```python
from build123d import *

# Parameters (mm, degrees)
EXTRUDE_1_DEPTH      = 12
CUT_EXTRUDE_1_DEPTH  = 12
SKETCH_3_R           = 2
CUT_EXTRUDE_2_DEPTH  = 12
CUT_EXTRUDE_3_DEPTH  = 1
SKETCH_5_W           = 80
SKETCH_5_H           = 4
CUT_EXTRUDE_4_DEPTH  = 20
EXTRUDE_2_DEPTH      = 1
SKETCH_7_W           = 0.2
SKETCH_7_H           = 8
CUT_EXTRUDE_5_DEPTH  = 1
SKETCH_8_R           = 2
EXTRUDE_3_DEPTH      = 4
SKETCH_9_W           = 80
SKETCH_9_H           = 9
CUT_EXTRUDE_6_DEPTH  = 14
SKETCH_10_W          = 9.44
SKETCH_10_H          = 1
CUT_EXTRUDE_7_DEPTH  = 14
SKETCH_11_W          = 9.44
SKETCH_11_H          = 1
EXTRUDE_4_DEPTH      = 8
CUT_EXTRUDE_8_DEPTH  = 8
SKETCH_13_W          = 80
SKETCH_13_H          = 3
EXTRUDE_5_DEPTH      = 7
SKETCH_14_R          = 1.6
EXTRUDE_7_DEPTH      = 3
SKETCH_16_W          = 3
SKETCH_16_H          = 4
EXTRUDE_8_DEPTH      = 80
SKETCH_17_R          = 1.55
CUT_EXTRUDE_11_DEPTH = 7
SKETCH_21_R          = 2
CUT_EXTRUDE_12_DEPTH = 7
EXTRUDE_9_DEPTH      = 4
SKETCH_23_W          = 3
SKETCH_23_H          = 4
CUT_EXTRUDE_13_DEPTH = 200
CUT_EXTRUDE_15_DEPTH = 5
SKETCH_25_W          = 9.44
SKETCH_25_H          = 4
CUT_EXTRUDE_16_DEPTH = 5
SKETCH_26_W          = 9.44
SKETCH_26_H          = 4
EXTRUDE_10_DEPTH     = 2
SKETCH_27_W          = 9.44
SKETCH_27_H          = 4
EXTRUDE_11_DEPTH     = 1
SKETCH_28_W          = 5
SKETCH_28_H          = 14
CUT_EXTRUDE_17_DEPTH = 1
SKETCH_29_W          = 5
SKETCH_29_H          = 4
EXTRUDE_12_DEPTH     = 1


with BuildPart() as part:
    # 草图1 → 凸台-拉伸1 (new body)
    with BuildSketch(Plane(origin=(0, 0, 0), x_dir=(1, 0, 0), z_dir=(0, 1, 0))):
        Polygon((-40, -6), (0, -6), (40, -6), (40, 0), (40, 6), (0, 6), (-36, 6), (-40, 6), align=None)
    extrude(amount=EXTRUDE_1_DEPTH)

    # 草图2 → 切除-拉伸1 (cut)
    with BuildSketch(Plane.XY.offset(6)):
        Polygon((-28, 0), (0, 0), (28, 0), (28, 4), (28, 8), (-28, 8), (-28, 4), align=None)
        Polygon((-40, 4), (-32, 4), (-32, 8), (-32, 12), (-40, 12), align=None)
        Polygon((32, 8), (32, 4), (40, 4), (40, 12), (32, 12), align=None)
    extrude(amount=-CUT_EXTRUDE_1_DEPTH, mode=Mode.SUBTRACT)

    # 草图3 → 切除-拉伸2 (cut)
    with BuildSketch(Plane(origin=(0, 12, 0), x_dir=(1, 0, 0), z_dir=(0, 1, 0))):
        with BuildLine():
            Line((-40, 6), (-40, 4))
            ThreePointArc((-40, 4), (-39.414213562, 5.414213562), (-38, 6))
            Line((-38, 6), (-40, 6))
        make_face()
        with Locations(Location((-36, 2, 0), (0, 0, 270))):
            Circle(SKETCH_3_R)
        with BuildLine():
            ThreePointArc((40, 4), (39.414213562, 5.414213562), (38, 6))
            Line((38, 6), (40, 6))
            Line((40, 6), (40, 4))
        make_face()
        with Locations(Location((36, 2, 0), (0, 0, 270))):
            Circle(SKETCH_3_R)
    extrude(amount=-CUT_EXTRUDE_2_DEPTH, mode=Mode.SUBTRACT)

    # 草图4 → 切除-拉伸3 (cut)
    with BuildSketch(Plane(origin=(0, 12, 0), x_dir=(1, 0, 0), z_dir=(0, 1, 0))):
        Polygon((-21.1, 0), (-21.1, 6), (-16.6, 6), (-12.1, 6), (12.08, 6), (16.6, 6), (21.12, 6), (21.12, -1), (21.12, -6), (16.6, -6), (12.08, -6), (12.08, -1), (12.08, 0), (-12.1, 0), (-12.1, -6), (-16.6, -6), (-21.1, -6), align=None)
    extrude(amount=-CUT_EXTRUDE_3_DEPTH, mode=Mode.SUBTRACT)

    # 草图5 → 切除-拉伸4 (cut)
    with BuildSketch(Plane(origin=(0, 12, 0), x_dir=(1, 0, 0), z_dir=(0, 1, 0))):
        with Locations((0, -4)):
            Rectangle(SKETCH_5_W, SKETCH_5_H)
    extrude(amount=-CUT_EXTRUDE_4_DEPTH, mode=Mode.SUBTRACT)

    # 草图6 → 凸台-拉伸2 (add)
    with BuildSketch(Plane(origin=(0, 12, 0), x_dir=(1, 0, 0), z_dir=(0, 1, 0))):
        Polygon((12.08, 0), (12.08, 6), (-21.1, 6), (-21.1, -2), (-12.1, -2), (-12.1, 0), align=None)
    extrude(amount=-EXTRUDE_2_DEPTH)

    # 草图7 → 切除-拉伸5 (cut)
    with BuildSketch(Plane(origin=(0, 12, 0), x_dir=(1, 0, 0), z_dir=(0, 1, 0))):
        with Locations((21.22, 2)):
            Rectangle(SKETCH_7_W, SKETCH_7_H)
        with Locations((11.98, 2)):
            Rectangle(SKETCH_7_W, SKETCH_7_H)
    extrude(amount=-CUT_EXTRUDE_5_DEPTH, mode=Mode.SUBTRACT)

    # 草图8 → 凸台-拉伸3 (add)
    # profile 1 of 2: a face of its own
    with BuildSketch(Plane(origin=(0, 12, 0), x_dir=(1, 0, 0), z_dir=(0, 1, 0))):
        with BuildLine():
            Line((-32, -2), (-40, -2))
            Line((-40, -2), (-40, 4))
            ThreePointArc((-40, 4), (-39.414213562, 5.414213562), (-38, 6))
            Line((-38, 6), (-32, 6))
            Line((-32, 6), (-32, -2))
        make_face()
        with Locations(Location((-36, 2, 0), (0, 0, 270))):
            Circle(SKETCH_8_R, mode=Mode.SUBTRACT)
    # profile 2 of 2: a face of its own
    with BuildSketch(Plane(origin=(0, 12, 0), x_dir=(1, 0, 0), z_dir=(0, 1, 0))):
        with BuildLine():
            Line((32, -2), (40, -2))
            Line((40, -2), (40, 4))
            ThreePointArc((40, 4), (39.414213562, 5.414213562), (38, 6))
            Line((38, 6), (32, 6))
            Line((32, 6), (32, -2))
        make_face()
        with Locations(Location((36, 2, 0), (0, 0, 270))):
            Circle(SKETCH_8_R, mode=Mode.SUBTRACT)
    extrude(amount=-EXTRUDE_3_DEPTH)

    # 草图9 → 切除-拉伸6 (cut)
    with BuildSketch(Plane.XY.offset(2)):
        with Locations((0, 4.5)):
            Rectangle(SKETCH_9_W, SKETCH_9_H)
    extrude(amount=-CUT_EXTRUDE_6_DEPTH, mode=Mode.SUBTRACT)

    # 草图10 → 切除-拉伸7 (cut)
    with BuildSketch(Plane(origin=(0, 0, -6), x_dir=(-1, 0, 0), z_dir=(0, 0, -1))):
        with Locations((-16.6, 9.5)):
            Rectangle(SKETCH_10_W, SKETCH_10_H)
    extrude(amount=-CUT_EXTRUDE_7_DEPTH, mode=Mode.SUBTRACT)

    # 草图11 → 凸台-拉伸4 (add)
    with BuildSketch(Plane(origin=(0, 0, -6), x_dir=(-1, 0, 0), z_dir=(0, 0, -1))):
        with Locations((-16.6, 11.5)):
            Rectangle(SKETCH_11_W, SKETCH_11_H)
    extrude(amount=-EXTRUDE_4_DEPTH)

    # 草图12 → 切除-拉伸8 (cut)
    with BuildSketch(Plane.XZ.offset(-9)):
        with BuildLine():
            ThreePointArc((21.05, -2.72), (18.302941274, 1.39126392), (13.453374824, 0.426625176))
            Line((13.453374824, 0.426625176), (19.746625176, -5.866625176))
            ThreePointArc((19.746625176, -5.866625176), (20.71126392, -4.422941274), (21.05, -2.72))
        make_face()
        with BuildLine():
            Line((19.746625176, -5.866625176), (13.453374824, 0.426625176))
            ThreePointArc((13.453374824, 0.426625176), (13.453374824, -5.866625176), (19.746625176, -5.866625176))
        make_face()
    extrude(amount=-CUT_EXTRUDE_8_DEPTH, mode=Mode.SUBTRACT)

    # 草图13 → 凸台-拉伸5 (add)
    with BuildSketch(Plane(origin=(0, 12, 0), x_dir=(1, 0, 0), z_dir=(0, 1, 0))):
        with Locations((0, -3.5)):
            Rectangle(SKETCH_13_W, SKETCH_13_H)
    extrude(amount=-EXTRUDE_5_DEPTH)

    # 草图14 → 凸台-拉伸7 (add)
    with BuildSketch(Plane(origin=(0, 12, 0), x_dir=(1, 0, 0), z_dir=(0, 1, 0))):
        with BuildLine():
            Line((-40, -100), (-40, -5))
            Line((-40, -5), (40, -5))
            Line((40, -5), (40, -100))
            Line((40, -100), (40, -102))
            ThreePointArc((40, -102), (39.414213562, -103.414213562), (38, -104))
            Line((38, -104), (36, -104))
            Line((36, -104), (-36, -104))
            Line((-36, -104), (-38, -104))
            ThreePointArc((-38, -104), (-39.414213562, -103.414213562), (-40, -102))
            Line((-40, -102), (-40, -100))
        make_face()
        with Locations(Location((-36, -100, 0), (0, 0, 270))):
            Circle(SKETCH_14_R, mode=Mode.SUBTRACT)
        with Locations(Location((36, -100, 0), (0, 0, 270))):
            Circle(SKETCH_14_R, mode=Mode.SUBTRACT)
    extrude(amount=-EXTRUDE_7_DEPTH)

    # 草图16 → 凸台-拉伸8 (add)
    with BuildSketch(Plane.ZY.offset(40)):
        with Locations((94.5, 7)):
            Rectangle(SKETCH_16_W, SKETCH_16_H)
    extrude(amount=-EXTRUDE_8_DEPTH)

    # 草图17 → 切除-拉伸11 (cut)
    with BuildSketch(Plane(origin=(0, 12, 0), x_dir=(1, 0, 0), z_dir=(0, 1, 0))):
        with Locations(Location((1.6, -34, 0), (0, 0, 270))):
            Circle(SKETCH_17_R)
        with Locations(Location((31.6, -34, 0), (0, 0, 270))):
            Circle(SKETCH_17_R)
        with Locations(Location((31.6, -64, 0), (0, 0, 270))):
            Circle(SKETCH_17_R)
        with Locations(Location((1.6, -64, 0), (0, 0, 270))):
            Circle(SKETCH_17_R)
    extrude(amount=-CUT_EXTRUDE_11_DEPTH, mode=Mode.SUBTRACT)

    # 草图21 → 切除-拉伸12 (cut)
    with BuildSketch(Plane(origin=(0, 12, 0), x_dir=(1, 0, 0), z_dir=(0, 1, 0))):
        with Locations(Location((-36, -100, 0), (0, 0, 270))):
            Circle(SKETCH_21_R)
        with Locations(Location((36, -100, 0), (0, 0, 270))):
            Circle(SKETCH_21_R)
    extrude(amount=-CUT_EXTRUDE_12_DEPTH, mode=Mode.SUBTRACT)

    # 草图22 → 凸台-拉伸9 (add)
    with BuildSketch(Plane(origin=(0, 9, 0), x_dir=(-1, 0, 0), z_dir=(0, -1, 0))):
        Polygon((40, -49), (40, -50.5), (-40, -50.5), (-40, -49), (-40, -47.5), (40, -47.5), align=None)
        Polygon((40, -26.25), (40, -27.75), (-40, -27.75), (-40, -24.75), (40, -24.75), align=None)
        Polygon((-40, -71.75), (-40, -73.25), (40, -73.25), (40, -70.25), (-40, -70.25), align=None)
    extrude(amount=EXTRUDE_9_DEPTH)

    # 草图23 → 切除-拉伸13 (cut)
    with BuildSketch(Plane.ZY.offset(40)):
        with Locations((3.5, 7)):
            Rectangle(SKETCH_23_W, SKETCH_23_H)
    extrude(amount=-CUT_EXTRUDE_13_DEPTH, mode=Mode.SUBTRACT)

    # 草图24 → 切除-拉伸15 (cut)
    with BuildSketch(Plane.XZ.offset(-9)):
        Polygon((11.88, -2), (11.88, 2), (16.6, 2), (16.6, 12), (9.6, 12), (9.6, -2), align=None)
        Polygon((16.6, 12), (16.6, 2), (21.32, 2), (21.32, -2), (23.6, -2), (23.6, 12), align=None)
    extrude(amount=-CUT_EXTRUDE_15_DEPTH, mode=Mode.SUBTRACT)

    # 草图25 → 切除-拉伸16 (cut)
    with BuildSketch(Plane(origin=(0, 10, 0), x_dir=(-1, 0, 0), z_dir=(0, -1, 0))):
        with Locations((-16.6, 0)):
            Rectangle(SKETCH_25_W, SKETCH_25_H)
    extrude(amount=-CUT_EXTRUDE_16_DEPTH, mode=Mode.SUBTRACT)

    # 草图26 → 凸台-拉伸10 (add)
    with BuildSketch(Plane(origin=(0, 10, 0), x_dir=(-1, 0, 0), z_dir=(0, -1, 0))):
        with Locations((-16.6, 4)):
            Rectangle(SKETCH_26_W, SKETCH_26_H)
    extrude(amount=-EXTRUDE_10_DEPTH)

    # 草图27 → 凸台-拉伸11 (add)
    with BuildSketch(Plane.XZ.offset(-10)):
        with Locations((16.6, -4)):
            Rectangle(SKETCH_27_W, SKETCH_27_H)
    extrude(amount=EXTRUDE_11_DEPTH)

    # 草图28 → 切除-拉伸17 (cut)
    with BuildSketch(Plane.XZ.offset(-9)):
        with Locations((7.1, 5)):
            Rectangle(SKETCH_28_W, SKETCH_28_H)
        with Locations((26.1, 5)):
            Rectangle(SKETCH_28_W, SKETCH_28_H)
    extrude(amount=-CUT_EXTRUDE_17_DEPTH, mode=Mode.SUBTRACT)

    # 草图29 → 凸台-拉伸12 (add)
    with BuildSketch(Plane.XZ.offset(-10)):
        with Locations((7.1, 0)):
            Rectangle(SKETCH_29_W, SKETCH_29_H)
        with Locations((26.1, 10)):
            Rectangle(SKETCH_29_W, SKETCH_29_H)
        with Locations((26.1, 0)):
            Rectangle(SKETCH_29_W, SKETCH_29_H)
        with Locations((7.1, 10)):
            Rectangle(SKETCH_29_W, SKETCH_29_H)
    extrude(amount=EXTRUDE_12_DEPTH)


solid = part.part
```
Check sheet for the modelled part. Datum: model origin and axes. Units: mm. A direction names the side the tool comes from. Give positions to 0.01 mm unless a question says otherwise; leave off trailing zeros. Order: outer loops, then holes, each group sorted by start corner. A loop starts at its lowest first (then second) coordinate and runs counter-clockwise, first axis right, second up. Notation, with made-up numbers: (13, 45) -> (45, 45) arc R7 cw to (45, 50) -> close; hole circle Ø9 at (33, 84.25). An arc over 180 degrees is marked (long way). Use CSV: the item, a comma, the result in double quotes. Start each with the question number.
1) Sectioned sample at B-B, the plane y = 7.5. Record the boundary of the cut face in (x, z), plus the area to 3 significant figures.
2) Set-up check for faces 1 (the face through (1, 9, 100)), 2 (the face through (-1, 7, 27.75)), 3 (the face through (26, 10, 5)), 4 (the face through (23.6, 11, 5)): record each of +Z, -Z, +X, -X, +Y, -Y from which the full face is reachable in a straight line by a thin tool's end or side.
3) Material ranges on line 1 (X direction, y = 10.75, z = 64); line 2 (X direction, y = 10.55, z = 100); line 3 (Z direction, x = -24, y = 6.25), recorded low to high. Write a range as from..to.
4) Mould release check, pull along Z, two halves, no side actions. Record for faces 5 (the face through (2.066, 10.521, 35.478)), 6 (the face through (-1, 11, -6)), 7 (the face through (1, 12, 48)): released by +Z, released by -Z, zero draft, split by the parting line, or undercut.
5) Sectioned sample at C-C, the plane x = 14.5. Record the boundary of the cut face in (y, z).
6) Sectioned sample at D-D, the plane x = 1.6. Record the boundary of the cut face in (y, z).
7) Sectioned sample at A-A, the plane z = 34. Record the boundary of the cut face in (x, y), plus the area to 3 significant figures.
8) Go/stop test with flat-tipped pins: P1, Ø1.2, axis at x = -14, y = 6.5, coming from the -Z side; P2, Ø10, axis at x = 11.5, z = 86.5, coming from the -Y side; P3, Ø3, axis at x = 10, y = 6.5, coming from the +Z side. Record where each tip stops, or that it passes through.
Recorded:
1,outline,"(-40, 24.75) -> (40, 24.75) -> (40, 27.75) -> (-40, 27.75) -> close; (-40, 47.5) -> (40, 47.5) -> (40, 50.5) -> (-40, 50.5) -> close; (-40, 70.25) -> (40, 70.25) -> (40, 73.25) -> (-40, 73.25) -> close; (-40, 93) -> (40, 93) -> (40, 96) -> (-40, 96) -> close"
1,area,"960 mm2"
2,face 1,"+Z, +X, -X, -Y"
2,face 2,"+X, -X, -Y"
2,face 3,"-Y"
2,face 4,"+Y, -Y"
3,line 1,"-40..0.05, 3.15..30.05, 33.15..40"
3,line 2,"-40..-38, -34..34, 38..40"
3,line 3,"24.75..27.75, 47.5..50.5, 70.25..73.25, 93..96"
4,face 5,"undercut"
4,face 6,"released by -Z"
4,face 7,"zero draft"
5,outline,"(5, 24.75) -> (9, 24.75) -> (9, 12) -> (12, 12) -> (12, 104) -> (9, 104) -> (9, 96) -> (5, 96) -> (5, 93) -> (9, 93) -> (9, 73.25) -> (5, 73.25) -> (5, 70.25) -> (9, 70.25) -> (9, 50.5) -> (5, 50.5) -> (5, 47.5) -> (9, 47.5) -> (9, 27.75) -> (5, 27.75) -> close; (9, -6) -> (12, -6) -> (12, -2) -> (9, -2) -> close"
6,outline,"(5, 24.75) -> (9, 24.75) -> (9, -6) -> (12, -6) -> (12, 32.45) -> (9, 32.45) -> (9, 27.75) -> (5, 27.75) -> close; (5, 47.5) -> (9, 47.5) -> (9, 35.55) -> (12, 35.55) -> (12, 62.45) -> (9, 62.45) -> (9, 50.5) -> (5, 50.5) -> close; (5, 70.25) -> (9, 70.25) -> (9, 65.55) -> (12, 65.55) -> (12, 104) -> (9, 104) -> (9, 96) -> (5, 96) -> (5, 93) -> (9, 93) -> (9, 73.25) -> (5, 73.25) -> close"
7,outline,"(-40, 9) -> (0.05, 9) -> (0.05, 12) -> (-40, 12) -> close; (3.15, 9) -> (30.05, 9) -> (30.05, 12) -> (3.15, 12) -> close; (33.15, 9) -> (40, 9) -> (40, 12) -> (33.15, 12) -> close"
7,area,"221 mm2"
8,P1,"z = 24.75"
8,P2,"y = 9"
8,P3,"z = 96"
